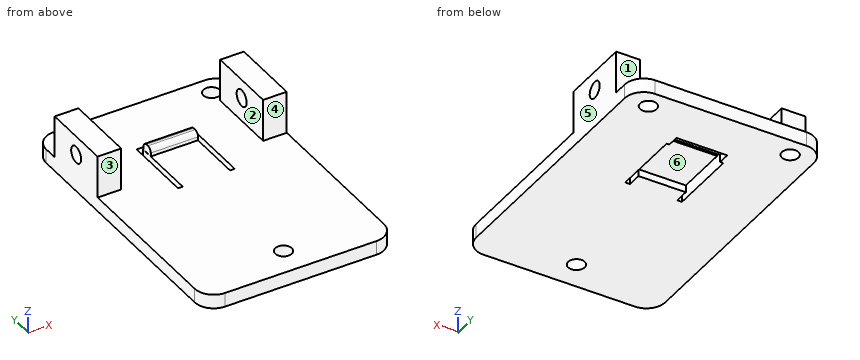
```python
from build123d import *

# Parameters (mm, degrees)
SKETCH_R        = 1.75
PAD_DEPTH       = 3
SKETCH001_W     = 10.76
SKETCH001_H     = 13.97
POCKET_DEPTH    = 1.5
SKETCH002_W     = 5
SKETCH002_H     = 15
PAD001_DEPTH    = 9
SKETCH003_R     = 1.75
POCKET001_DEPTH = 50
SKETCH004_W     = 10
SKETCH004_H     = 2.5
PAD002_DEPTH    = 1.75
FILLET_R        = 1


with BuildPart() as part:
    # Sketch → Pad (new body)
    with BuildSketch(Plane.XY):
        with BuildLine():
            Line((-20, -26), (-20, 26))
            ThreePointArc((-20, 26), (-18.828427, 28.828427), (-16, 30))
            Line((-16, 30), (16, 30))
            ThreePointArc((16, 30), (18.828427, 28.828427), (20, 26))
            Line((20, 26), (20, -26))
            ThreePointArc((20, -26), (18.828427, -28.828427), (16, -30))
            Line((16, -30), (-16, -30))
            ThreePointArc((-16, -30), (-18.828427, -28.828427), (-20, -26))
        make_face()
        Polygon((6, 3), (5, 3), (5, 17), (-5, 17), (-5, 3), (-6, 3), (-6, 17.5), (6, 17.5), align=None, mode=Mode.SUBTRACT)
        with Locations((-15, 26)):
            Circle(SKETCH_R, mode=Mode.SUBTRACT)
        with Locations((15, 26)):
            Circle(SKETCH_R, mode=Mode.SUBTRACT)
        with Locations((0, -24)):
            Circle(SKETCH_R, mode=Mode.SUBTRACT)
    extrude(amount=PAD_DEPTH)

    # Sketch001 → Pocket (cut)
    with BuildSketch(Plane.XY):
        with Locations((0.05, 12.985)):
            Rectangle(SKETCH001_W, SKETCH001_H)
    extrude(amount=POCKET_DEPTH, mode=Mode.SUBTRACT)

    # Sketch002 → Pad001 (join)
    with BuildSketch(Plane.XY.offset(3)):
        with Locations((17.5, 15.5)):
            Rectangle(SKETCH002_W, SKETCH002_H)
        with Locations((-17.5, 15.5)):
            Rectangle(SKETCH002_W, SKETCH002_H)
    extrude(amount=PAD001_DEPTH)

    # Sketch003 → Pocket001 (cut)
    with BuildSketch(Plane.YZ.offset(20)):
        with Locations((15.5, 8)):
            Circle(SKETCH003_R)
    extrude(amount=-POCKET001_DEPTH, mode=Mode.SUBTRACT)

    # Sketch004 → Pad002 (join)
    with BuildSketch(Plane.XY.offset(3)):
        with Locations((0.024575, 15.5)):
            Rectangle(SKETCH004_W, SKETCH004_H)
    extrude(amount=PAD002_DEPTH)

    # Fillet
    fillet_edges = [part.edges().sort_by_distance(p)[0] for p in [
        (0.024575, 14.25, 4.75),
        (0.024575, 16.75, 4.75),
    ]]
    fillet(fillet_edges, radius=FILLET_R)


solid = part.part
```
Model file for the job. Use its own axes, mm. Face numbers are marked on the shaded views. A direction names the side the tool comes from. Give positions to 0.01 mm unless a question says otherwise; leave off trailing zeros. Loops run counter-clockwise (first coordinate to the right, second up) from the corner with the lowest first, then second, coordinate; pieces in that order, holes last. Notation, with made-up numbers: (87.5, -1.5) -> (124.5, -1.5) arc R24 cw to (124.5, 11.5) -> close; hole circle Ø11 at (60, 26.25). An arc over 180 degrees is marked (long way). Use CSV: the item, a comma, the result in double quotes. Start each with the question number.
1) Flat gauge pins, fed straight in: pin 1 Ø10 at (x, y) = (-10.5, -5) entering from +Z; pin 2 Ø3 at (x, y) = (-0.5, 11) entering from -Z; pin 3 Ø2.5 at (x, z) = (-17.5, 8.5) entering from -Y. Where does each tip first touch, or does it go through?
2) Wall check: line 1 (Y direction, x = 0, z = 1.4); line 2 (X direction, y = 20, z = 4.5); line 3 (Y direction, x = -15, z = 1.9). Give the ranges that are in metal, low to high.
3) Mould opens along X. For the marked faces 4, 5 and 6 say: released by +X, released by -X, zero draft, split by the parting line, or undercut.
4) Slice it at B-B on x = 0. Give the cut face in (y, z).
5) Slice it at D-D on y = -12.5. Give the cut face in (x, z).
6) Tool access for the marked faces 1, 2 and 3: list every direction of +Z, -Z, +X, -X, +Y, -Y with a clear straight run to the whole face (end or side of a thin tool).
7) Slice it at A-A on z = 8. Give the cut face in (x, y), plus the area to 3 significant figures.
8) Slice it at C-C on y = -23. Give the cut face in (x, z), plus the area to 3 significant figures.
Computed values:
1,pin 1,"stops at z = 3"
1,pin 2,"stops at z = 1.5"
1,pin 3,"stops at y = 8"
2,line 1,"y = -30 to -25.75, -22.25 to 6, 19.97 to 30"
2,line 2,"x = -20 to -15, 15 to 20"
2,line 3,"y = -30 to 24.25, 27.75 to 30"
3,face 4,"zero draft"
3,face 5,"released by +X"
3,face 6,"undercut"
4,outline,"(-30, 0) -> (-25.75, 0) -> (-25.75, 3) -> (-30, 3) -> close; (-22.25, 0) -> (6, 0) -> (6, 1.5) -> (17, 1.5) -> (17, 3) -> (16.75, 3) -> (16.75, 3.75) arc R1 ccw to (15.75, 4.75) -> (15.25, 4.75) arc R1 ccw to (14.25, 3.75) -> (14.25, 3) -> (-22.25, 3) -> close; (17.5, 1.5) -> (19.97, 1.5) -> (19.97, 0) -> (30, 0) -> (30, 3) -> (17.5, 3) -> close"
5,outline,"(-20, 0) -> (20, 0) -> (20, 3) -> (-20, 3) -> close"
6,face 1,"+Z, +X, -X, +Y"
6,face 2,"+Z, +Y, -Y"
6,face 3,"+Z, +X, -X, -Y"
7,outline,"(-20, 8) -> (-15, 8) -> (-15, 13.75) -> (-20, 13.75) -> close; (-20, 17.25) -> (-15, 17.25) -> (-15, 23) -> (-20, 23) -> close; (15, 8) -> (20, 8) -> (20, 13.75) -> (15, 13.75) -> close; (15, 17.25) -> (20, 17.25) -> (20, 23) -> (15, 23) -> close"
7,area,"115 mm^2"
8,outline,"(-20, 0) -> (-1.44, 0) -> (-1.44, 3) -> (-20, 3) -> close; (1.44, 0) -> (20, 0) -> (20, 3) -> (1.44, 3) -> close"
8,area,"111 mm^2"
